from build123d import *

# Parameters (mm, degrees)
F0_W     = 200
F0_H     = 200
F1_DEPTH = 10
F3_R     = 15
F4_DEPTH = 10.001
F5_R     = 40
F6_SIZE2 = 110
F6_SIZE  = 80


with BuildPart() as f1:
    # F0 (on Front) → F1 (new body)
    with BuildSketch(Plane.XZ):
        Rectangle(F0_W, F0_H)
    extrude(amount=-F1_DEPTH)

    # F3 (on face) → F4 (cut, through all)
    with BuildSketch(Plane.XZ):
        with Locations((-55, -55)):
            Circle(F3_R)
        with Locations((55, 55)):
            Circle(F3_R)
    extrude(amount=-F4_DEPTH, mode=Mode.SUBTRACT)

    # F5
    f5_edges = [f1.edges().sort_by_distance(p)[0] for p in [
        (-100, 5, -100),
    ]]
    fillet(f5_edges, radius=F5_R)

    # F6
    f6_edges = [f1.edges().sort_by_distance(p)[0] for p in [
        (-100, 5, 100),
    ]]
    f6_side = f1.faces().sort_by_distance((0, 5, 100))[0]
    chamfer(f6_edges, length=F6_SIZE, length2=F6_SIZE2, reference=f6_side)


solid = f1.part
Check sheet for the modelled part. Datum: model origin and axes. Units: mm. Round coordinates to 2 decimals unless told otherwise and drop trailing zeros. Loops run counter-clockwise (first coordinate to the right, second up) from the corner with the lowest first, then second, coordinate; pieces in that order, holes last. Notation, with made-up numbers: M 23,68 L 55,68 A18 cw 55,89 Z; hole C -34,31 d7. An arc over 180 degrees is marked long. One line per item, written item: value.
(1) Sectioned sample at A-A, the plane z = -55. Record the cut outline in (x, y), then the cut area to 3 significant figures.
Computed values:
outline: M -100,0 L -70,0 L -70,10 L -100,10 Z; M -40,0 L 100,0 L 100,10 L -40,10 Z
area: 1,700 mm^2
(2) Sectioned sample at D-D, the plane z = 24.5. Record the cut outline in (x, y).
Computed values:
outline: M -74.91,0 L 100,0 L 100,10 L -74.91,10 Z
(3) Depth check by flat-ended pin: pin 1 Ø18 at (x, z) = (-55, -55) entering from -Y; pin 2 Ø4 at (y, z) = (3.5, 78.5) entering from -X; pin 3 Ø2 at (y, z) = (6.5, -80) entering from -X. Enter the tip coordinate at first touch or a pass-through.
Computed values:
pin 1: passes through
pin 2: stops at x = -37.09
pin 3: stops at x = -95.2
(4) Thickness scan on line 1 (Z direction, x = 55, y = 2.75); line 2 (Z direction, x = 66.5, y = 1.25); line 3 (X direction, y = 3.25, z = -42.5). Record the ranges inside material, lowest first.
Computed values:
line 1: z = -100 to 40, 70 to 100
line 2: z = -100 to 45.37, 64.63 to 100
line 3: x = -100 to -63.29, -46.71 to 100
(5) Release check for a two-part mould opening along Z. For faces 1 (the face through (40.015, 4.93, 55.66)), 2 (the face through (19, 5, -100)), 3 (the face through (100, 5, -1)) record: +Z half, -Z half, draft (parallel to the pull), parting line (faces both ways), or undercut.
Computed values:
face 1: undercut
face 2: -Z half
face 3: draft
(6) Sectioned sample at C-C, the plane y = 4. Record the cut outline in (x, z).
Computed values:
outline: M -100,-60 A40 ccw -60,-100 L 100,-100 L 100,100 L -20,100 L -100,-10 Z; hole C -55,-55 d30; hole C 55,55 d30
(7) Sectioned sample at B-B, the plane x = 61.5. Record the cut outline in (y, z), then the cut area to 3 significant figures.
Computed values:
outline: M 0,-100 L 10,-100 L 10,41.48 L 0,41.48 Z; M 0,68.52 L 10,68.52 L 10,100 L 0,100 Z
area: 1,730 mm^2
